Input: part model. Units: mm. Frame: model coordinates. A direction names the side the tool comes from. Round coordinates to 2 decimals unless told otherwise and drop trailing zeros. Loops run counter-clockwise (first coordinate to the right, second up) from the corner with the lowest first, then second, coordinate; pieces in that order, holes last.
1) First-contact query: pin 1 (3 mm diameter, centred on x = 29.5, z = 9, fed in from -Y); pin 2 (1 mm diameter, centred on y = 127, z = -128.5, fed in from +X); pin 3 (5 mm diameter, centred on x = 12.5, z = 4.5, fed in from +Y). Flat tips, straight axial feed; report the tip coordinate or a pass-through.
2) Section A-A, the plane y = 73. Return loops of the section in (x, z).
3) Ray query, line 1 along X through (y, z) = (83, -40.5); line 2 along Y through (x, z) = (56.5, -126); line 3 along Z through (x, y) = (45, 210). Return the intervals inside material, ascending.
4) Draft query along X for faces 1 (the face through (-62.99, 115.86, 95.72)), 2 (the face through (64.5, 117, -9)), 3 (the face through (67.5, 116, -9)). Return one class per face: pulls with the +X half, pulls with the -X half, needs draft (parallel to the pull), parting line crosses it, or undercut.
5) Section C-C, the plane z = 19.5. Return loops of the section in (x, y), and give its area (3 significant figures).
6) Access query for faces 4 (the face through (-1.418, 117.376, -164.484)), 5 (the face through (-67.5, 116, -6)). Directions: +Z, -Z, +X, -X, +Y, -Y. A direction counts if a zero-diameter tool reaches every point of the face in a straight line with its end or side. Return the directions, or none.
7) Section B-B, the plane x = 0. Return loops of the section in (y, z), and give its area (3 significant figures).
from build123d import *

# Parameters (mm, degrees)
BOSS_EXTRUDE1_DEPTH = 235
SHELL1_T            = -3


with BuildPart() as part:
    # Sketch1 → Boss-Extrude1 (new body)
    with BuildSketch(Plane(origin=(0, 0, 0), x_dir=(1, 0, 0), z_dir=(0, 1, 0))):
        with BuildLine():
            Line((52.5, -100), (-52.5, -100))
            ThreePointArc((-52.5, -100), (-63.106601718, -95.606601718), (-67.5, -85))
            Line((-67.5, -85), (-67.5, 100))
            ThreePointArc((-67.5, 100), (0, 167.5), (67.5, 100))
            Line((67.5, 100), (67.5, -85))
            ThreePointArc((67.5, -85), (63.106601718, -95.606601718), (52.5, -100))
        make_face()
    extrude(amount=BOSS_EXTRUDE1_DEPTH)

    # Shell1
    shell1_openings = [part.faces().sort_by_distance(p)[0] for p in [
        (0, 235, 18.118867239),
    ]]
    offset(amount=SHELL1_T, openings=shell1_openings, kind=Kind.INTERSECTION)


solid = part.part
Final values:
1. pin 1: stops at y = 0
1. pin 2: stops at x = 61.42
1. pin 3: stops at y = 3
2. outline: (-67.5, -100) arc R67.5 ccw to (67.5, -100) - (67.5, 85) arc R15 ccw to (52.5, 100) - (-52.5, 100) arc R15 ccw to (-67.5, 85) - close; hole (-64.5, -100) arc R64.5 ccw to (64.5, -100) - (64.5, 85) arc R12 ccw to (52.5, 97) - (-52.5, 97) arc R12 ccw to (-64.5, 85) - close
3. line 1: x = -67.5 to -64.5, 64.5 to 67.5
3. line 2: y = 0 to 3
3. line 3: z = -150.31 to -146.21, 97 to 100
4. face 1: pulls with the -X half
4. face 2: undercut
4. face 3: pulls with the +X half
5. outline: (-67.5, 0) - (67.5, 0) - (67.5, 235) - (64.5, 235) - (64.5, 3) - (-64.5, 3) - (-64.5, 235) - (-67.5, 235) - close
5. area: 1,800 mm2
6. face 4: +Y
6. face 5: +Z, -Z, -X, +Y, -Y
7. outline: (0, -167.5) - (235, -167.5) - (235, -164.5) - (3, -164.5) - (3, 97) - (235, 97) - (235, 100) - (0, 100) - close
7. area: 2,190 mm2
